from build123d import *

# Parameters (mm, degrees)
BOX024_W     = 150
BOX024_H     = 37
BOX024_DEPTH = 45
BOX023_W     = 150
BOX023_H     = 37
BOX023_DEPTH = 45


with BuildPart() as obj1:
    # Box024 → Box024 (new body)
    with BuildSketch(Plane(origin=(-3, 0, 3), x_dir=(1, 0, 0), z_dir=(0, 0, 1))):
        with Locations((75, 18.5)):
            Rectangle(BOX024_W, BOX024_H)
    extrude(amount=BOX024_DEPTH)


with BuildPart() as cut018:
    # Box023 → Box023 (new body)
    with BuildSketch(Plane.XY):
        with Locations((75, 18.5)):
            Rectangle(BOX023_W, BOX023_H)
    extrude(amount=BOX023_DEPTH)

    # Cut018: cut obj1
    add(obj1.part, mode=Mode.SUBTRACT)


with BuildPart() as cut018_1:
    # Cut018 placement: moved
    add(cut018.part.moved(Location((10, 30, 0))))


solid = cut018_1.part
Read the model definition and answer for the solid it produces. Units are mm, in the model's axes. A direction names the side the tool comes from. Round coordinates to 2 decimals unless told otherwise and drop trailing zeros. Order: outer loops, then holes, each group sorted by start corner. A loop starts at its lowest first (then second) coordinate and runs counter-clockwise, first axis right, second up. Notation, with made-up numbers: (76.25, 32) - (106.25, 32) arc R19 cw to (106.25, 48) - close; hole circle Ø6 at (33, 77). An arc over 180 degrees is marked (long way). Use one line per item in the form item = value. Start each with the question number.
(1) For faces 1 (the face through (85, 67, 1)), 2 (the face through (82, 49, 3)), determine the directions among +Z, -Z, +X, -X, +Y, -Y from which every point of the face is accessible in a straight line to the end or side of a thin tool.
(2) The part is cut by section C-C (z = 28). Give the vertices of the cut face in (x, y), then the cut area to 3 significant figures.
(3) The part is cut by section B-B (x = 127). Give the vertices of the cut face in (y, z).
(4) Find the intervals of material crossed by line 1 along X through (y, z) = (59.5, 12.5); line 2 along Z through (x, y) = (114.5, 52.5), in increasing order. Write a range as from..to.
(5) The part is cut by section A-A (y = 50.5). Give the vertices of the cut face in (x, z).
(6) Flat-ended cylindrical pins translate along their axes: pin 1 Ø4 at (y, z) = (59, 14) entering from -X; pin 2 Ø5 at (x, y) = (66, 36.5) entering from +Z. Find the tip coordinate at first contact, or state that the pin passes through.
Checked values:
q1.face_1 = +Z, -Z, +X, -X, +Y
q1.face_2 = +Z, -X, +Y, -Y
q2.outline = (157, 30) - (160, 30) - (160, 67) - (157, 67) - close
q2.area = 111 mm^2
q3.outline = (30, 0) - (67, 0) - (67, 3) - (30, 3) - close
q4.line_1 = 157..160
q4.line_2 = 0..3
q5.outline = (10, 0) - (160, 0) - (160, 45) - (157, 45) - (157, 3) - (10, 3) - close
q6.pin_1 = 157
q6.pin_2 = 3
